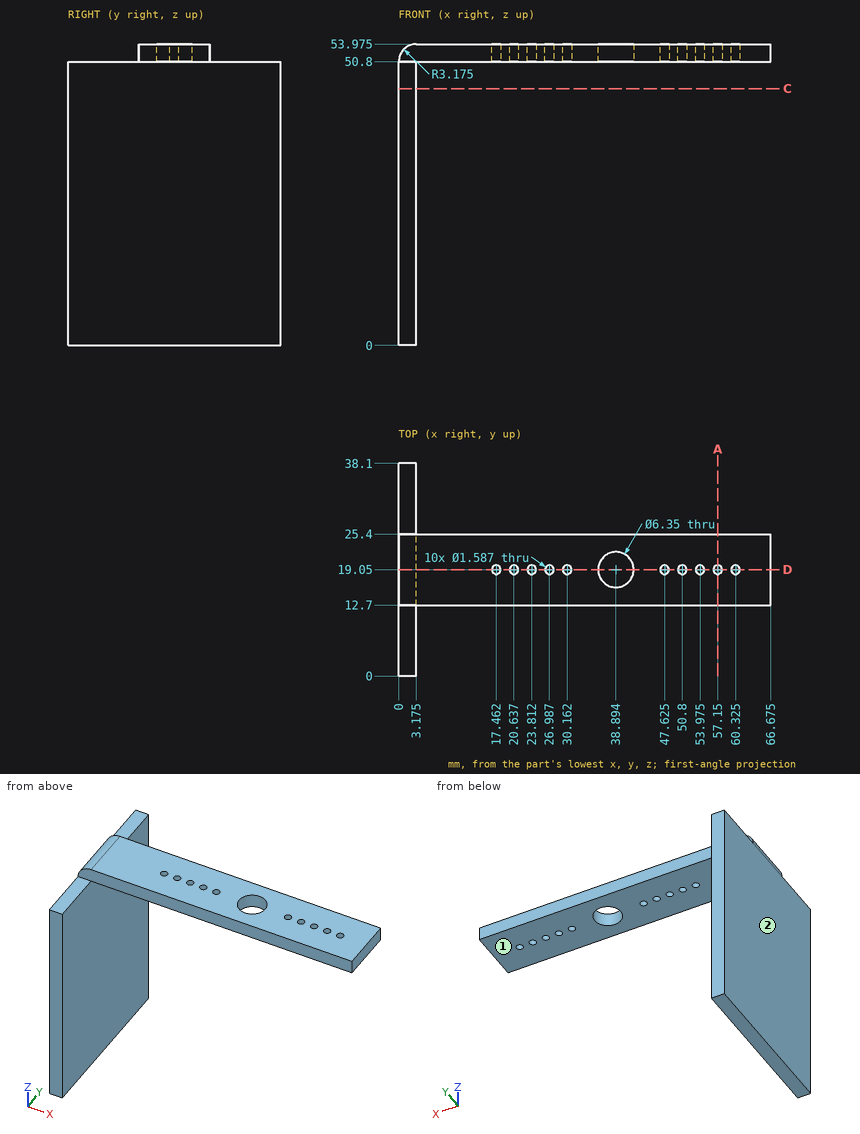
Study the drawing (mm; zero at the part's minimum x, y, z) and answer. A direction names the side the tool comes from. Round coordinates to 2 decimals unless told otherwise and drop trailing zeros. Write each loop counter-clockwise with the first axis right and the second up, starting at its lowest first coordinate (ties: lowest second). Pieces come first, ordered by that corner, then holes.
Q1. A tool of negligible diameter and unlimited length cuts with its end or side. For the marked faces 1 and 2, from which of +Z, -Z, +X, -X, +Y, -Y can it reach the whole face along a straight path? Write none if from no direction.
Values:
face 1: -Z, +X, +Y, -Y
face 2: +Z, -Z, -X, +Y, -Y
Q2. Straight lines are drawn through the part: line 1 (Y direction, x = 57.15, z = 51.5); line 2 (X direction, y = 13, z = 22.5) (1 decimal); line 3 (Z direction, x = 29, y = 20) (1 decimal). For each, find the intervals that lie inside material, in ascending order.
Values:
line 1: y = 12.7 to 18.26, 19.84 to 25.4
line 2: x = 0 to 3.2
line 3: z = 50.8 to 54
Q3. Find section A-A on x = 57.15. Determine the outline of the cut face in (y, z) (1 decimal).
Values:
outline: (12.7, 50.8) - (18.3, 50.8) - (18.3, 54) - (12.7, 54) - close; (19.8, 50.8) - (25.4, 50.8) - (25.4, 54) - (19.8, 54) - close
Q4. Flat-ended cylindrical pins translate along their axes: P1, Ø8, axis at x = 37.5, y = 9, coming from the -Z side; P2, Ø2, axis at x = 50.8, y = 19.05, coming from the +Z side (1 decimal); P3, Ø1.6, axis at x = 33.5, z = 52, coming from the +Y side; P4, Ø1.6, axis at x = 45, z = 51.5, coming from the -Y side. Find the tip coordinate at first contact, or state that the pin passes through.
Values:
P1: stops at z = 50.8
P2: stops at z = 54
P3: stops at y = 25.4
P4: stops at y = 12.7
Q5. Find section D-D on y = 19.05. State how many separate pieces and enclosed holes the cut face has.
Values:
separate pieces: 12
enclosed holes: 0
Q6. Find section C-C on z = 46. Determine the outline of the cut face in (x, y) (1 decimal), and give its area (3 significant figures).
Values:
outline: (0, 0) - (3.2, 0) - (3.2, 38.1) - (0, 38.1) - close
area: 121 mm2
